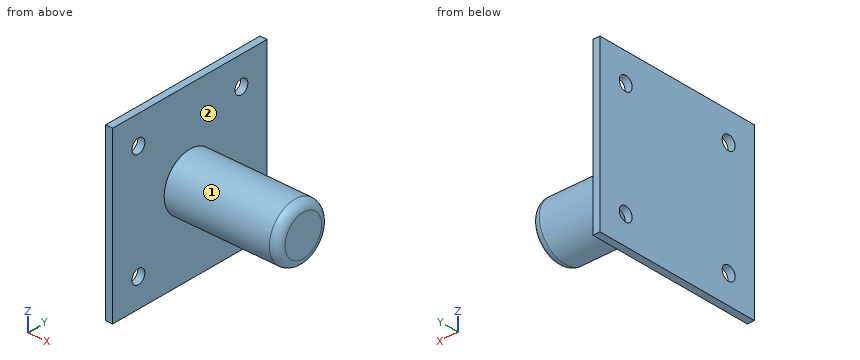
```python
from build123d import *

# Parameters (mm, degrees)
SKETCH1_W           = 76.2
SKETCH1_H           = 76.2
SKETCH1_R           = 3.175
BOSS_EXTRUDE1_DEPTH = 1.5875


with BuildPart() as part:
    # Sketch1 → Boss-Extrude1 (new, symmetric)
    with BuildSketch(Plane(origin=(0, 0, 0), x_dir=(0, 0, -1), z_dir=(1, 0, 0))):
        Rectangle(SKETCH1_W, SKETCH1_H)
        with Locations((-25.4, 25.4)):
            Circle(SKETCH1_R, mode=Mode.SUBTRACT)
        with Locations((25.4, 25.4)):
            Circle(SKETCH1_R, mode=Mode.SUBTRACT)
        with Locations((25.4, -25.4)):
            Circle(SKETCH1_R, mode=Mode.SUBTRACT)
        with Locations((-25.4, -25.4)):
            Circle(SKETCH1_R, mode=Mode.SUBTRACT)
    extrude(amount=BOSS_EXTRUDE1_DEPTH, both=True)

    # Sketch2 → Revolve1 (revolve)
    with BuildSketch(Plane.XY, mode=Mode.PRIVATE) as revolve1_sk:
        with BuildLine():
            Line((48.70420202, 12.7), (1.5875, 12.7))
            Line((1.5875, 12.7), (1.5875, 0))
            Line((1.5875, 0), (52.3875, 0))
            Line((52.3875, 0), (52.3875, 9.01670202))
            ThreePointArc((52.3875, 9.01670202), (51.308686999, 11.621186999), (48.70420202, 12.7))
        make_face()
    revolve(revolve1_sk.sketch.rotate(Axis((1.5875, 0, 0), (1, 0, 0)), 90), axis=Axis((1.5875, 0, 0), (1, 0, 0)))


solid = part.part
```
Can you work these out from the model? Positions are in its coordinate system, mm. Face numbers are marked on the shaded views. Round coordinates to 2 decimals unless told otherwise and drop trailing zeros. Loops run counter-clockwise (first coordinate to the right, second up) from the corner with the lowest first, then second, coordinate; pieces in that order, holes last. Notation, with made-up numbers: M 3,6.5 L 7,6.5 A23 ccw 7,38.5 Z; hole C 45.25,80.25 d1. An arc over 180 degrees is marked long. Answer as a JSON object with one key per item and string values. Group by question number.
Q1. Will these pins go through, and if not, where does the flat tip stop? pin 1 (4 mm diameter, centred on x = 40, y = -6.5, fed in from +Z); pin 2 (8 mm diameter, centred on x = 12.5, z = 3.5, fed in from +Y); pin 3 (8 mm diameter, centred on y = 13.5, z = 14.5, fed in from +X).
Q2. Imagine slicing it at B-B, the plane y = 27. Please give me the cut outline in (x, z).
Q3. Imagine slicing it at D-D, the plane x = 16.5. Please give me the cut outline in (y, z).
Q4. Imagine slicing it at A-A, the plane z = -25.4. Please give me the cut outline in (x, y) (1 decimal).
Q5. We'd pull the mould along Y, two halves only. Please class the marked faces 1 and 2: +Y half, -Y half, draft (parallel to the pull), parting line (faces both ways), or undercut.
Q6. Imagine slicing it at C-C, the plane y = 0. Please give me the cut outline in (x, z).
Q7. Please list where these lines run through material, in increasing order: L1, parallel to Y at x = -0.45, z = 25.4 (3 decimals); L2, parallel to Z at x = 0, y = -25.
Findings:
{
 "1": {"pin 1": "stops at z = 11.88", "pin 2": "stops at y = 12.7", "pin 3": "stops at x = 1.59"},
 "2": {"outline": "M -1.59,-38.1 L 1.59,-38.1 L 1.59,-28.14 L -1.59,-28.14 Z; M -1.59,-22.66 L 1.59,-22.66 L 1.59,22.66 L -1.59,22.66 Z; M -1.59,28.14 L 1.59,28.14 L 1.59,38.1 L -1.59,38.1 Z"},
 "3": {"outline": "C 0,0 d25.4"},
 "4": {"outline": "M -1.6,-38.1 L 1.6,-38.1 L 1.6,-28.6 L -1.6,-28.6 Z; M -1.6,-22.2 L 1.6,-22.2 L 1.6,22.2 L -1.6,22.2 Z; M -1.6,28.6 L 1.6,28.6 L 1.6,38.1 L -1.6,38.1 Z"},
 "5": {"face 1": "parting line", "face 2": "draft"},
 "6": {"outline": "M -1.59,-38.1 L 1.59,-38.1 L 1.59,-12.7 L 48.7,-12.7 A3.68 ccw 52.39,-9.02 L 52.39,9.02 A3.68 ccw 48.7,12.7 L 1.59,12.7 L 1.59,38.1 L -1.59,38.1 Z"},
 "7": {"L1": "y = -38.1 to -28.575, -22.225 to 22.225, 28.575 to 38.1", "L2": "z = -38.1 to -28.55, -22.25 to 22.25, 28.55 to 38.1"}
}
